Could you check a few things on this model? Use its own coordinates, in mm. A direction names the side the tool comes from. Coordinates: 2 decimals unless noted, no trailing zeros. Loops run counter-clockwise (first coordinate to the right, second up) from the corner with the lowest first, then second, coordinate; pieces in that order, holes last.
1) If I drill on line 1 along Y through (x, z) = (30, 21.15); line 2 along X through (y, z) = (40, 20.85); line 3 along X through (y, z) = (-25, 21.25), over which ranges is the centre line in solid material (lowest first)?
2) Will these pins go through, and if not, where does the flat tip stop? P1, Ø25, axis at x = -4, y = 5, coming from the +Z side; P2, Ø2, axis at y = 2, z = 18.5, coming from the -X side; P3, Ø1.5, axis at x = 8, y = -32.5, coming from the -Z side.
3) Imagine slicing it at B-B on y = 40. Please give me the cut outline in (x, z).
4) Thinking about a two-plate mould opening in Y: for faces 4 (the face through (0, 31.35, 19)), 5 (the face through (-25, 8, 18)), 6 (the face through (19.367, -10.967, 22.014)), 7 (the face through (0, -30, 18)), which applies, released by +Y, released by -Y, zero draft, split by the parting line, or undercut?
5) Imagine slicing it at D-D on y = -16.5. Please give me the cut outline in (x, z), plus the area to 3 significant figures.
6) Imagine slicing it at C-C on z = 18.05. Please give me the cut outline in (x, y) (3 decimals).
7) Imagine slicing it at A-A on x = -30. Please give me the cut outline in (y, z).
8) For faces 1 (the face through (35, 1, 21)), 2 (the face through (-20.354, -10.587, 22.014)), 3 (the face through (13.437, 30.598, 19.028)), which set-ups out of +Z, -Z, +X, -X, +Y, -Y let a thin tool reach every point of the face, with its end or its side?
Autodesk Inventor part; units mm, degrees
ref_plane "YZ Plane" through (0, 0, 0) normal (1, 0, 0) x (0, 1, 0)
ref_plane "XZ Plane" through (0, 0, 0) normal (0, 1, 0) x (-1, 0, 0)
ref_plane "XY Plane" through (0, 0, 0) normal (0, 0, 1) x (1, 0, 0)
sketch "Sketch1" plane through (0, 0, 0) normal (0, 0, 1) x (1, 0, 0)
  line L0 (-35, 45) -> (35, 45)
  line L1 (35, 45) -> (35, -45)
  line L2 (35, -45) -> (-35, -45)
  line L3 (-35, -45) -> (-35, 45)
  point P0 (0, 0)
  point P1 (0, 45)
  point P2 (-35, 0)
  dimension "d0" = 70
  dimension "d1" = 90
extrude "Extrusion1" add sketch "Sketch1" along normal blind 23
sketch "Sketch2" plane through (0, 0, 23) normal (0, 0, 1) x (1, 0, 0)
  circle A0 centre (-20.425, 3.625) radius 3.15
  circle A1 centre (19.575, 3.625) radius 3.15
  line L0 (12.1727, -25.475) -> (-13.0227, -25.475)
  arc A2 (-14.903, -24.1567) -> (-13.0227, -25.475) centre (-13.0227, -23.475) ccw
  line L1 (-14.903, -24.1567) -> (-24.7279, 2.9433)
  arc A3 (-24.7279, 4.3067) -> (-24.7279, 2.9433) centre (-22.8476, 3.625) ccw
  line L2 (-24.7279, 4.3067) -> (-14.903, 31.4067)
  arc A4 (-13.0227, 32.725) -> (-14.903, 31.4067) centre (-13.0227, 30.725) ccw
  line L3 (-13.0227, 32.725) -> (12.1727, 32.725)
  arc A5 (14.053, 31.4067) -> (12.1727, 32.725) centre (12.1727, 30.725) ccw
  line L4 (14.053, 31.4067) -> (23.8779, 4.3067)
  arc A6 (23.8779, 2.9433) -> (23.8779, 4.3067) centre (21.9976, 3.625) ccw
  line L5 (23.8779, 2.9433) -> (14.053, -24.1567)
  arc A7 (12.1727, -25.475) -> (14.053, -24.1567) centre (12.1727, -23.475) ccw
  line L6 (-12.5, 30.85) -> (11.65, 30.85)
  arc A8 (13.65, 28.85) -> (11.65, 30.85) centre (11.65, 28.85) ccw
  line L7 (13.65, 28.85) -> (13.65, -21.6)
  arc A9 (11.65, -23.6) -> (13.65, -21.6) centre (11.65, -21.6) ccw
  line L8 (11.65, -23.6) -> (-12.5, -23.6)
  arc A10 (-14.5, -21.6) -> (-12.5, -23.6) centre (-12.5, -21.6) ccw
  line L9 (-14.5, -21.6) -> (-14.5, 28.85)
  arc A11 (-12.5, 30.85) -> (-14.5, 28.85) centre (-12.5, 28.85) ccw
  line L10 (11.875, -14) -> (11.875, -4.28)
  arc A12 (11.875, -4.28) -> (9.875, -2.28) centre (9.875, -4.28) ccw
  line L11 (9.875, -2.28) -> (-10.725, -2.28)
  arc A13 (-10.725, -2.28) -> (-12.725, -4.28) centre (-10.725, -4.28) ccw
  line L12 (-12.725, -4.28) -> (-12.725, -14)
  line L13 (-12.725, -14) -> (-7.725, -19)
  line L14 (-7.725, -19) -> (6.875, -19)
  line L15 (6.875, -19) -> (11.875, -14)
  line L16 (0.575, -12.25) -> (0.575, -15.75)
  line L17 (0.575, -15.75) -> (-1.425, -15.75)
  line L18 (-1.425, -15.75) -> (-1.425, -12.25)
  line L19 (-1.425, -12.25) -> (0.575, -12.25)
  line L20 (-6.3111, -5.53) -> (-6.3111, -9.03)
  line L21 (-6.3111, -9.03) -> (-8.3111, -9.03)
  line L22 (-8.3111, -9.03) -> (-8.3111, -5.53)
  line L23 (-8.3111, -5.53) -> (-6.3111, -5.53)
  line L24 (5.4611, -9.03) -> (5.4611, -5.53)
  line L25 (5.4611, -5.53) -> (7.4611, -5.53)
  line L26 (7.4611, -5.53) -> (7.4611, -9.03)
  line L27 (7.4611, -9.03) -> (5.4611, -9.03)
  line L28 (11.65, 31.35) -> (-12.5, 31.35)
  arc A14 (-12.5, 31.35) -> (-15, 28.85) centre (-12.5, 28.85) ccw
  line L29 (-15, 28.85) -> (-15, -21.6)
  arc A15 (-15, -21.6) -> (-12.5, -24.1) centre (-12.5, -21.6) ccw
  line L30 (-12.5, -24.1) -> (11.65, -24.1)
  arc A16 (11.65, -24.1) -> (14.15, -21.6) centre (11.65, -21.6) ccw
  line L31 (14.15, -21.6) -> (14.15, 28.85)
  arc A17 (14.15, 28.85) -> (11.65, 31.35) centre (11.65, 28.85) ccw
  dimension "d90" = 0.5
extrude "Extrusion2" cut sketch "Sketch2" against normal through all contours L6 A8 L7 A9 L8 A10 L9 A11 | L15 L14 L13 L12 A13 L11 A12 L10 | L16 L17 L18 L19 | L20 L21 L22 L23 | L24 L25 L26 L27 | A17 L31 A16 L30 A15 L29 A14 L28
sketch "Sketch3" plane through (0, 0, 23) normal (0, 0, 1) x (1, 0, 0)
  circle A0 centre (-20.425, 3.625) radius 3.15
  circle A1 centre (19.575, 3.625) radius 3.15
  line L0 (12.1727, -25.475) -> (-13.0227, -25.475)
  arc A2 (-14.903, -24.1567) -> (-13.0227, -25.475) centre (-13.0227, -23.475) ccw
  line L1 (-14.903, -24.1567) -> (-24.7279, 2.9433)
  arc A3 (-24.7279, 4.3067) -> (-24.7279, 2.9433) centre (-22.8476, 3.625) ccw
  line L2 (-24.7279, 4.3067) -> (-14.903, 31.4067)
  arc A4 (-13.0227, 32.725) -> (-14.903, 31.4067) centre (-13.0227, 30.725) ccw
  line L3 (-13.0227, 32.725) -> (12.1727, 32.725)
  arc A5 (14.053, 31.4067) -> (12.1727, 32.725) centre (12.1727, 30.725) ccw
  line L4 (14.053, 31.4067) -> (23.8779, 4.3067)
  arc A6 (23.8779, 2.9433) -> (23.8779, 4.3067) centre (21.9976, 3.625) ccw
  line L5 (23.8779, 2.9433) -> (14.053, -24.1567)
  arc A7 (12.1727, -25.475) -> (14.053, -24.1567) centre (12.1727, -23.475) ccw
  line L6 (-12.5, 30.85) -> (11.65, 30.85)
  arc A8 (13.65, 28.85) -> (11.65, 30.85) centre (11.65, 28.85) ccw
  line L7 (13.65, 28.85) -> (13.65, -21.6)
  arc A9 (11.65, -23.6) -> (13.65, -21.6) centre (11.65, -21.6) ccw
  line L8 (11.65, -23.6) -> (-12.5, -23.6)
  arc A10 (-14.5, -21.6) -> (-12.5, -23.6) centre (-12.5, -21.6) ccw
  line L9 (-14.5, -21.6) -> (-14.5, 28.85)
  arc A11 (-12.5, 30.85) -> (-14.5, 28.85) centre (-12.5, 28.85) ccw
  line L10 (11.875, -14) -> (11.875, -4.28)
  arc A12 (11.875, -4.28) -> (9.875, -2.28) centre (9.875, -4.28) ccw
  line L11 (9.875, -2.28) -> (-10.725, -2.28)
  arc A13 (-10.725, -2.28) -> (-12.725, -4.28) centre (-10.725, -4.28) ccw
  line L12 (-12.725, -4.28) -> (-12.725, -14)
  line L13 (-12.725, -14) -> (-7.725, -19)
  line L14 (-7.725, -19) -> (6.875, -19)
  line L15 (6.875, -19) -> (11.875, -14)
  line L16 (0.575, -12.25) -> (0.575, -15.75)
  line L17 (0.575, -15.75) -> (-1.425, -15.75)
  line L18 (-1.425, -15.75) -> (-1.425, -12.25)
  line L19 (-1.425, -12.25) -> (0.575, -12.25)
  line L20 (-6.3111, -5.53) -> (-6.3111, -9.03)
  line L21 (-6.3111, -9.03) -> (-8.3111, -9.03)
  line L22 (-8.3111, -9.03) -> (-8.3111, -5.53)
  line L23 (-8.3111, -5.53) -> (-6.3111, -5.53)
  line L24 (5.4611, -9.03) -> (5.4611, -5.53)
  line L25 (5.4611, -5.53) -> (7.4611, -5.53)
  line L26 (7.4611, -5.53) -> (7.4611, -9.03)
  line L27 (7.4611, -9.03) -> (5.4611, -9.03)
  line L28 (12.1727, 33.225) -> (-13.0227, 33.225)
  arc A14 (-13.0227, 33.225) -> (-15.373, 31.5771) centre (-13.0227, 30.725) ccw
  line L29 (-15.373, 31.5771) -> (-25.1979, 4.4771)
  arc A15 (-25.1979, 4.4771) -> (-25.1979, 2.7729) centre (-22.8476, 3.625) ccw
  line L30 (-25.1979, 2.7729) -> (-15.373, -24.3271)
  arc A16 (-15.373, -24.3271) -> (-13.0227, -25.975) centre (-13.0227, -23.475) ccw
  line L31 (-13.0227, -25.975) -> (12.1727, -25.975)
  arc A17 (12.1727, -25.975) -> (14.523, -24.3271) centre (12.1727, -23.475) ccw
  line L32 (14.523, -24.3271) -> (24.3479, 2.7729)
  arc A18 (24.3479, 2.7729) -> (24.3479, 4.4771) centre (21.9976, 3.625) ccw
  line L33 (24.3479, 4.4771) -> (14.523, 31.5771)
  arc A19 (14.523, 31.5771) -> (12.1727, 33.225) centre (12.1727, 30.725) ccw
  dimension "d91" = 0.5
extrude "Extrusion3" cut sketch "Sketch3" against normal blind 2 contours A0 | A1 | L0 A2 L1 A3 L2 A4 L3 A5 L4 A6 L5 A7 | L6 A8 L7 A9 L8 A10 L9 A11 | L15 L14 L13 L12 A13 L11 A12 L10 | L16 L17 L18 L19 | L20 L21 L22 L23 | L24 L25 L26 L27 | A19 L33 A18 L32 A17 L31 A16 L30 A15 L29 A14 L28
sketch "Sketch4" plane through (0, 0, 0) normal (0, 0, -1) x (-1, 0, 0)
  line L0 (-25, 45) -> (25, 45)
  line L1 (25, 45) -> (25, -30)
  line L2 (25, -30) -> (-25, -30)
  line L3 (-25, -30) -> (-25, 45)
  line L4 (-35, -45) -> (-35, 45)
  line L5 (35, -45) -> (-35, -45)
  line L6 (-35, 45) -> (35, 45)
  line L7 (35, 45) -> (35, -45)
  point P0 (0, 0)
  point P1 (45, -30)
  point P2 (-25, 45)
  point P3 (0, -30)
  point P4 (0, -45)
  point P5 (25, 45)
  dimension "d11" = 15
  dimension "d89" = 10
extrude "Extrusion4" cut sketch "Sketch4" against normal blind 20 contours L3 L2 L1 L6 L7 L5 L4
sketch "Sketch6" plane through (0, 0, 23) normal (0, 0, 1) x (1, 0, 0)
  circle A0 centre (-19.865, 3.655) radius 1.6
  circle A1 centre (20.135, 3.655) radius 1.6
  point P0 (0, 0)
hole "Hole1" at (20.135, 3.655, 23) at (-19.865, 3.655, 23) direction (0, 0, -1) diameter 4 end through all
sketch "Sketch5" plane through (0, 0, 0) normal (0, 0, -1) x (-1, 0, 0)
  line L0 (-20, 45) -> (45, 45)
  line L1 (-20, 0) -> (-20, 45)
  line L2 (-25, 45) -> (35, 45)
  line L3 (-25, 45) -> (-25, -30)
  line L4 (-25, -30) -> (25, -30)
  line L5 (14.9072, -25) -> (34.9072, -25)
  line L6 (35, -30) -> (14.9072, -30)
  line L7 (14.9072, -25) -> (14.9072, -30)
  line L8 (-25, 0) -> (-20, 0)
  line L9 (35, 45) -> (35, -30)
  point P0 (-20, -30)
  point P1 (14.9072, -30)
  point P2 (-20, 45)
  point P3 (14.9072, -30)
  point P4 (35, 45)
  dimension "d17" = 5
  dimension "d35" = 5
  dimension "d80" = 30
  dimension "d96" = 20.0928
extrude "Extrusion5" cut sketch "Sketch5" against normal blind 17
sketch "Sketch9" plane through (0, 0, 17) normal (0, 0, -1) x (-1, 0, 0)
  line L0 (-25, 45) -> (25, 45)
  line L1 (25, -30) -> (-25, -30)
  line L2 (-9.15, -24.1) -> (20, -24.1)
  line L3 (20, -24.1) -> (20, -30)
  line L4 (20, -30) -> (-9.15, -30)
  line L5 (-9.15, -30) -> (-9.15, -24.1)
  line L6 (-25, -30) -> (-25, 45)
  line L7 (25, 45) -> (25, -30)
  line L8 (-14.15, 28.85) -> (-14.15, -21.6)
  arc A0 (-11.65, 31.35) -> (-14.15, 28.85) centre (-11.65, 28.85) ccw
  line L9 (12.5, 31.35) -> (-11.65, 31.35)
  arc A1 (15, 28.85) -> (12.5, 31.35) centre (12.5, 28.85) ccw
  line L10 (15, -21.6) -> (15, 28.85)
  arc A2 (12.5, -24.1) -> (15, -21.6) centre (12.5, -21.6) ccw
  line L11 (-11.65, -24.1) -> (12.5, -24.1)
  arc A3 (-14.15, -21.6) -> (-11.65, -24.1) centre (-11.65, -21.6) ccw
  point P0 (0, 0)
  point P1 (-9.15, -30)
  point P2 (20, -30)
extrude "Extrusion6" [suppressed]
sketch "Sketch10" plane through (-17.5, -24.1, 21) normal (0, 1, 0) x (1, 0, 0)
  line L0 (22.5, 19) -> (2.5, 19)
  line L1 (2.5, 19) -> (2.5, 29)
  line L2 (2.5, 29) -> (22.5, 29)
  line L3 (22.5, 29) -> (22.5, 19)
  point P0 (17.5, 21)
  point P1 (12.5, 29)
  point P2 (12.5, 34)
  dimension "d94" = 10
extrude "Extrusion7" [suppressed]
fillet "Fillet1" [suppressed]
sketch "Sketch11" plane through (0, 0, 23) normal (0, 0, 1) x (1, 0, 0)
  line L0 (-35, -45) -> (35, -45)
  line L1 (-35, 45) -> (-35, -45)
  line L2 (35, -45) -> (35, 45)
  line L3 (35, 45) -> (-35, 45)
  point P0 (0, 0)
  point P1 (-15, -40)
  point P2 (15, -40)
  point P3 (30, -25)
  point P4 (30, 40)
  point P5 (-30, 40)
  point P6 (-30, -25)
  dimension "d65" = 5
  dimension "d66" = 20
  dimension "d67" = 20
  dimension "d68" = 5
  dimension "d69" = 5
  dimension "d70" = 20
  dimension "d71" = 5
  dimension "d72" = 5
  dimension "d97" = 5
hole "Hole4" at (-15, -40, 23) at (15, -40, 23) at (30, -25, 23) at (30, 40, 23) at (-30, 40, 23) at (-30, -25, 23) direction (0, 0, -1) diameter 4 end through all countersink diameter 7 countersink angle 90
chamfer "Chamfer2" distance 2 angle 45 4 edges at (-35, 45, 21.5) (35, 45, 21.5) (35, -45, 21.5) (-35, -45, 21.5)
properties part number "10-06-015 Suport conector cablu"
Filled in:
1. line 1: y = -45 to -27, -23 to 38, 42 to 45
1. line 2: x = -35 to -32, -28 to 28, 32 to 35
1. line 3: x = -35 to -32, -28 to -15, 14.15 to 28, 32 to 35
2. P1: stops at z = 21
2. P2: stops at x = -25
2. P3: stops at z = 20
3. outline: (-35, 20) - (-32, 20) - (-32, 21.5) - (-33.5, 23) - (-35, 23) - close; (-28, 20) - (-25, 20) - (-25, 17) - (25, 17) - (25, 20) - (28, 20) - (28, 21.5) - (26.5, 23) - (-26.5, 23) - (-28, 21.5) - close; (32, 20) - (35, 20) - (35, 23) - (33.5, 23) - (32, 21.5) - close
4. face 4: undercut
4. face 5: zero draft
4. face 6: undercut
4. face 7: released by -Y
5. outline: (-35, 20) - (-25, 20) - (-25, 17) - (-15, 17) - (-15, 21) - (-18.21, 21) - (-18.21, 23) - (-35, 23) - close; (14.15, 17) - (25, 17) - (25, 20) - (35, 20) - (35, 23) - (17.36, 23) - (17.36, 21) - (14.15, 21) - close
5. area: 172 mm2
6. outline: (-25, -30) - (25, -30) - (25, 45) - (-25, 45) - close; hole circle Ø4 at (-19.865, 3.655); hole (-15, -21.6) arc R2.5 ccw to (-12.5, -24.1) - (11.65, -24.1) arc R2.5 ccw to (14.15, -21.6) - (14.15, 28.85) arc R2.5 ccw to (11.65, 31.35) - (-12.5, 31.35) arc R2.5 ccw to (-15, 28.85) - close; hole circle Ø4 at (20.135, 3.655)
7. outline: (-45, 20) - (-27, 20) - (-27, 21.5) - (-28.5, 23) - (-45, 23) - close; (-23, 20) - (38, 20) - (38, 21.5) - (36.5, 23) - (-21.5, 23) - (-23, 21.5) - close; (42, 20) - (45, 20) - (45, 23) - (43.5, 23) - (42, 21.5) - close
8. face 1: +Z, -Z, +X, +Y, -Y
8. face 2: +Z
8. face 3: +Z, -Z
